```python
from build123d import *

# Parameters (mm, degrees)
BOSS_EXTRUDE1_DEPTH     = 25
BOSS_EXTRUDE2_START     = 25
SKETCH1_3_R             = 22.5
BOSS_EXTRUDE2_DEPTH     = 15
BOSS_EXTRUDE2_TAPER     = 15
SKETCH4_R               = 27.5
CUT_EXTRUDE3_DEPTH      = 8
SKETCH1_4_R             = 10
CUT_EXTRUDE1_DEPTH      = 124.288280092
CUT_EXTRUDE2_DEPTH      = 124.288280092
CUT_EXTRUDE2_DEPTH_BACK = 124.288280092


with BuildPart() as part:
    # Sketch1 → Boss-Extrude1 (new body)
    with BuildSketch(Plane(origin=(0, 0, 0), x_dir=(1, 0, 0), z_dir=(0, 1, 0))):
        with BuildLine():
            Line((-90, -60), (90, -60))
            ThreePointArc((90, -60), (97.071067812, -57.071067812), (100, -50))
            Line((100, -50), (100, -32))
            Line((100, -32), (50, -32))
            ThreePointArc((50, -32), (42.928932188, -29.071067812), (40, -22))
            Line((40, -22), (40, 22))
            ThreePointArc((40, 22), (42.928932188, 29.071067812), (50, 32))
            Line((50, 32), (100, 32))
            Line((100, 32), (100, 50))
            ThreePointArc((100, 50), (97.071067812, 57.071067812), (90, 60))
            Line((90, 60), (-90, 60))
            ThreePointArc((-90, 60), (-97.071067812, 57.071067812), (-100, 50))
            Line((-100, 50), (-100, 32))
            Line((-100, 32), (-50, 32))
            ThreePointArc((-50, 32), (-42.928932188, 29.071067812), (-40, 22))
            Line((-40, 22), (-40, -22))
            ThreePointArc((-40, -22), (-42.928932188, -29.071067812), (-50, -32))
            Line((-50, -32), (-100, -32))
            Line((-100, -32), (-100, -50))
            ThreePointArc((-100, -50), (-97.071067812, -57.071067812), (-90, -60))
        make_face()
    extrude(amount=BOSS_EXTRUDE1_DEPTH)

    # Sketch1<3> → Boss-Extrude2 (add)
    with BuildSketch(Plane(origin=(0, 0, 0), x_dir=(1, 0, 0), z_dir=(0, 1, 0)).offset(BOSS_EXTRUDE2_START)):
        Circle(SKETCH1_3_R)
    extrude(amount=BOSS_EXTRUDE2_DEPTH, taper=BOSS_EXTRUDE2_TAPER)

    # Sketch4 → Cut-Extrude3 (cut)
    with BuildSketch(Plane(origin=(0, 25, 0), x_dir=(1, 0, 0), z_dir=(0, 1, 0))):
        with BuildLine():
            Line((-95, 50), (-95, 37))
            Line((-95, 37), (-50, 37))
            ThreePointArc((-50, 37), (-39.393398282, 32.606601718), (-35, 22))
            Line((-35, 22), (-35, -22))
            ThreePointArc((-35, -22), (-39.393398282, -32.606601718), (-50, -37))
            Line((-50, -37), (-95, -37))
            Line((-95, -37), (-95, -50))
            ThreePointArc((-95, -50), (-93.535533906, -53.535533906), (-90, -55))
            Line((-90, -55), (90, -55))
            ThreePointArc((90, -55), (93.535533906, -53.535533906), (95, -50))
            Line((95, -50), (95, -37))
            Line((95, -37), (50, -37))
            ThreePointArc((50, -37), (39.393398282, -32.606601718), (35, -22))
            Line((35, -22), (35, 22))
            ThreePointArc((35, 22), (39.393398282, 32.606601718), (50, 37))
            Line((50, 37), (95, 37))
            Line((95, 37), (95, 50))
            ThreePointArc((95, 50), (93.535533906, 53.535533906), (90, 55))
            Line((90, 55), (-90, 55))
            ThreePointArc((-90, 55), (-93.535533906, 53.535533906), (-95, 50))
        make_face()
        with Locations(Location((0, 0, 0), (0, 0, 270))):
            Circle(SKETCH4_R, mode=Mode.SUBTRACT)
    extrude(amount=-CUT_EXTRUDE3_DEPTH, mode=Mode.SUBTRACT)

    # Sketch1<4> → Cut-Extrude1 (cut, through all)
    with BuildSketch(Plane(origin=(0, 0, 0), x_dir=(1, 0, 0), z_dir=(0, 1, 0))):
        with Locations(Location((0, 0, 0), (0, 0, 270))):
            Circle(SKETCH1_4_R)
    extrude(amount=CUT_EXTRUDE1_DEPTH, mode=Mode.SUBTRACT)

    # Sketch3 → Cut-Extrude2 (cut, two sides: drawn at the far end of the back side and taken through both)
    with BuildSketch(Plane.XY.offset(-CUT_EXTRUDE2_DEPTH_BACK)):
        Polygon((40, 25), (100, 12.5), (100, 25), align=None)
    extrude(amount=CUT_EXTRUDE2_DEPTH + CUT_EXTRUDE2_DEPTH_BACK, mode=Mode.SUBTRACT)


solid = part.part
```
Work out the finished part from the listing and answer in its coordinate system (mm). A direction names the side the tool comes from. Give positions to 0.01 mm unless a question says otherwise; leave off trailing zeros. Order: outer loops, then holes, each group sorted by start corner. A loop starts at its lowest first (then second) coordinate and runs counter-clockwise, first axis right, second up.
1. Section C-C, the plane x = -29.5 is taken. Determine the outline of the cut face in (y, z).
Result sheet:
outline: (0, -60) - (25, -60) - (25, -55) - (17, -55) - (17, 55) - (25, 55) - (25, 60) - (0, 60) - close
2. Each of these flat-tipped pins is pushed along its axis until it touches: P1, Ø10, axis at y = 15.5, z = -4.5, coming from the -X side; P2, Ø6.5, axis at y = 20, z = -3, coming from the +X side; P3, Ø1.5, axis at x = 37.5, z = -7.5, coming from the +Y side; P4, Ø4, axis at x = 76, z = 40, coming from the -Y side. Where does it stop, or does it pass through?
Result sheet:
P1: stops at x = -40
P2: stops at x = 40
P3: stops at y = 25
P4: stops at y = 0
3. Section D-D, the plane x = 45 is taken. Determine the outline of the cut face in (y, z).
Result sheet:
outline: (0, -60) - (23.96, -60) - (23.96, -55) - (17, -55) - (17, -36.14) - (23.96, -36.14) - (23.96, -30.66) - (0, -30.66) - close; (0, 30.66) - (23.96, 30.66) - (23.96, 36.14) - (17, 36.14) - (17, 55) - (23.96, 55) - (23.96, 60) - (0, 60) - close
4. The mould has two halves that part along X. Classify faces 4 (the flat face through (-36, 25, 0)), 5 (the flat face through (-40, 12, 0)), 6 (the flat face through (35, 21, 0)): released by +X, released by -X, zero draft, split by the parting line, or undercut.
Result sheet:
face 4: zero draft
face 5: released by -X
face 6: undercut
5. Section A-A, the plane y = 9.5 is taken. Determine the outline of the cut face in (x, z).
Result sheet:
outline: (-100, -50) arc R10 ccw to (-90, -60) - (90, -60) arc R10 ccw to (100, -50) - (100, -32) - (50, -32) arc R10 cw to (40, -22) - (40, 22) arc R10 cw to (50, 32) - (100, 32) - (100, 50) arc R10 ccw to (90, 60) - (-90, 60) arc R10 ccw to (-100, 50) - (-100, 32) - (-50, 32) arc R10 cw to (-40, 22) - (-40, -22) arc R10 cw to (-50, -32) - (-100, -32) - close; hole circle Ø20 at (0, 0)
6. For faces 1 (the flat face through (58, 19, -37)), 2 (the cylindrical face through (-42.85, 12.32, 28.99)), 3 (the flat face through (-29, 17, -1)), determine the directions among +Z, -Z, +X, -X, +Y, -Y from which every point of the face is accessible in a straight line to the end or side of a thin tool.
Result sheet:
face 1: +X, +Y
face 2: -X, +Y, -Y
face 3: +Y
7. Straight lines are drawn through the part: L1, parallel to X at y = 22, z = 0; L2, parallel to Z at x = -82, y = 8; L3, parallel to X at y = 11, z = 0. For each, find the intervals that lie inside material, in ascending order.
Result sheet:
L1: x = -40 to -35, -27.5 to -10, 10 to 27.5, 35 to 40
L2: z = -60 to -32, 32 to 60
L3: x = -40 to -10, 10 to 40
8. Section B-B, the plane x = 0 is taken. Determine the outline of the cut face in (y, z), and give its area (3 significant figures).
Result sheet:
outline: (0, -60) - (25, -60) - (25, -55) - (17, -55) - (17, -27.5) - (25, -27.5) - (25, -22.5) - (40, -18.48) - (40, -10) - (0, -10) - close; (0, 10) - (40, 10) - (40, 18.48) - (25, 22.5) - (25, 27.5) - (17, 27.5) - (17, 55) - (25, 55) - (25, 60) - (0, 60) - close
area: 2,370 mm2
